Build history of the part. All positions in model axes, mm. Face numbers are marked on the shaded views. A direction names the side the tool comes from. Round coordinates to 2 decimals unless told otherwise and drop trailing zeros. Write each loop counter-clockwise with the first axis right and the second up, starting at its lowest first coordinate (ties: lowest second). Pieces come first, ordered by that corner, then holes. Notation, with made-up numbers: M 45,34.25 L 98,34.25 A29 ccw 98,58.25 Z; hole C 14,-22 d2. An arc over 180 degrees is marked long. One line per item, written item: value. Start each with the question number.
```python
from build123d import *

# Parameters (mm, degrees)
SKETCH1_R           = 20.5
BOSS_EXTRUDE1_DEPTH = 2
SKETCH2_R           = 5.15
CUT_EXTRUDE1_DEPTH  = 3
SKETCH3_R           = 6.5
CUT_EXTRUDE2_DEPTH  = 2
BOSS_EXTRUDE4_DEPTH = 30


with BuildPart() as part:
    # Sketch1 → Boss-Extrude1 (new body)
    with BuildSketch(Plane(origin=(0, 0, 0), x_dir=(1, 0, 0), z_dir=(0, 1, 0))):
        with Locations(Location((0, 0, 0), (0, 0, 270))):
            Circle(SKETCH1_R)
    extrude(amount=BOSS_EXTRUDE1_DEPTH)

    # Sketch2 → Cut-Extrude1 (cut)
    with BuildSketch(Plane(origin=(0, 2, 0), x_dir=(1, 0, 0), z_dir=(0, 1, 0))):
        with Locations(Location((0, 0, 0), (0, 0, 270))):
            Circle(SKETCH2_R)
    extrude(amount=-CUT_EXTRUDE1_DEPTH, mode=Mode.SUBTRACT)

    # Sketch3 → Cut-Extrude2 (cut)
    with BuildSketch(Plane(origin=(0, 2, 0), x_dir=(1, 0, 0), z_dir=(0, 1, 0))):
        with Locations(Location((0, 13, 0), (0, 0, 270))):
            Circle(SKETCH3_R)
    extrude(amount=-CUT_EXTRUDE2_DEPTH, mode=Mode.SUBTRACT)

    # Sketch4 → Boss-Extrude4 (add)
    with BuildSketch(Plane(origin=(0, 2, 0), x_dir=(1, 0, 0), z_dir=(0, 1, 0))):
        with BuildLine():
            Line((-16.620770139, 12), (-3.5, 5.5))
            Line((-3.5, 5.5), (3.5, 5.5))
            Line((3.5, 5.5), (16.620770139, 12))
            ThreePointArc((16.620770139, 12), (13.206287248, 15.679412525), (9, 18.418740456))
            ThreePointArc((9, 18.418740456), (0, 5.93152382), (-9, 18.418740456))
            ThreePointArc((-9, 18.418740456), (-13.206287248, 15.679412525), (-16.620770139, 12))
        make_face()
    extrude(amount=BOSS_EXTRUDE4_DEPTH)


solid = part.part
```
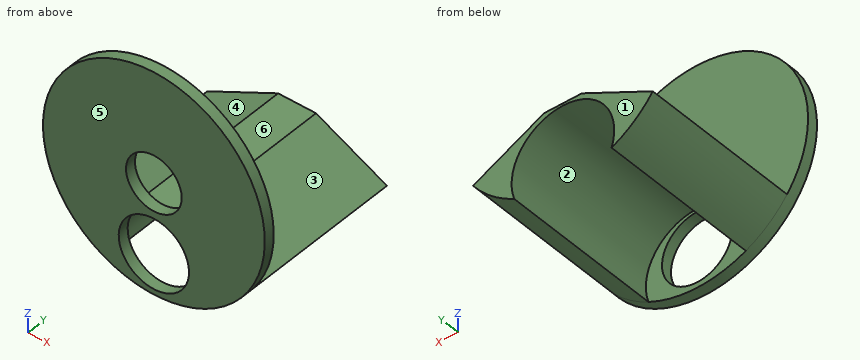
Item 1: Cut at B-B, the plane x = 0. Write the cut outline in (y, z).
Item 2: Cut at A-A, the plane z = 0. Write the cut outline in (x, y), plus the area to 3 significant figures.
Item 3: Cut at C-C, the plane y = 14. Write the cut outline in (x, z).
Item 4: Two-plate mould, pull along X, no slides. Class the marked faces 1, 2 and 3: pulls with the +X half, pulls with the -X half, needs draft (parallel to the pull), parting line crosses it, or undercut.
Item 5: Which spindle directions (+Z, -Z, +X, -X, +Y, -Y) get a long thin tool onto all of the face, cutting with end or side? Do the marked faces 4, 5 and 6. Say none if no direction does.
Item 6: Drop flat-ended pins along their axis: pin 1 (11.5 mm diameter, centred on x = 0, z = -13, fed in from +Y); pin 2 (3.5 mm diameter, centred on x = 0, y = 23, fed in from +Z); pin 3 (10 mm diameter, centred on x = 2.5, z = 4.5, fed in from +Y); pin 4 (6 mm diameter, centred on y = 20.5, z = -5, fed in from -X). Give the stop position or say it passes through.
Item 7: Cut at D-D, the plane z = -13. Write the cut outline in (x, y).
Item 8: Drill centre lines: line 1 (X direction, y = 1.65, z = 0); line 2 (Y direction, x = 8, z = -0.5); line 3 (Z direction, x = 0, y = 16). Where is each one in solid material? Low to high.
Computed values:
1. outline: M 0,-20.5 L 2,-20.5 L 2,-19.5 L 0,-19.5 Z; M 0,-6.5 L 2,-6.5 L 2,-5.93 L 32,-5.93 L 32,-5.5 L 2,-5.5 L 2,-5.15 L 0,-5.15 Z; M 0,5.15 L 2,5.15 L 2,20.5 L 0,20.5 Z
2. outline: M -20.5,0 L -5.15,0 L -5.15,2 L -20.5,2 Z; M 5.15,0 L 20.5,0 L 20.5,2 L 5.15,2 Z
2. area: 61.4 mm2
3. outline: M -16.62,-12 A20.5 ccw -9,-18.42 A9.49 cw long 9,-18.42 A20.5 ccw 16.62,-12 L 3.5,-5.5 L -3.5,-5.5 Z
4. face 1: needs draft
4. face 2: undercut
4. face 3: pulls with the +X half
5. face 4: +Z, -X, +Y
5. face 5: +Z, -Z, +X, -X, -Y
5. face 6: +Z, +X, -X, +Y
6. pin 1: passes through
6. pin 2: stops at z = -5.5
6. pin 3: stops at y = 2
6. pin 4: stops at x = -8.55
7. outline: M -15.85,0 L -6.5,0 L -6.5,2 L -9.17,2 L -9.17,32 L -15.85,32 Z; M 6.5,0 L 15.85,0 L 15.85,32 L 9.17,32 L 9.17,2 L 6.5,2 Z
8. line 1: x = -20.5 to -5.15, 5.15 to 20.5
8. line 2: y = 0 to 2
8. line 3: z = -5.93 to -5.5
